Print and shaded views of the part. All mm, measured from the part's lowest x, y and z. A direction names the side the tool comes from. Coordinates: 2 decimals unless noted, no trailing zeros. Loops run counter-clockwise (first coordinate to the right, second up) from the corner with the lowest first, then second, coordinate; pieces in that order, holes last. Notation, with made-up numbers: (14, -2) -> (52, -2) arc R22 ccw to (52, 11) -> close; hole circle Ø7 at (13, 2.5). An arc over 180 degrees is marked (long way). One line per question, with ' | ' between items. Start each with the question number.
1) Probe L1, parallel to Y at x = 9.75, z = 8.5; L2, parallel to Y at x = 1.5, z = 3; L3, parallel to Z at x = 12.25, y = 17.5. List the from-to ranges inside material, lowest first. Write a range as from..to.
2) Cut at A-A (x = 7.05). List the corners of the cut face in (y, z), plus the area to 3 significant figures.
3) Drop flat-ended pins along their axis: pin 1 (2 mm diameter, centred on x = 3, y = 22.5, fed in from +Z); pin 2 (1.5 mm diameter, centred on y = 29, z = 1.5, fed in from +X); pin 3 (4 mm diameter, centred on x = 3.5, y = 34, fed in from +Z). Give the stop position or say it passes through.
4) 3-axis set-ups, long thin cutter, end or side, ignore diameter. For the marked faces 1 and 2: which of +Z, -Z, +X, -X, +Y, -Y reach the whole face in a straight line?
5) Cut at B-B (y = 17). List the corners of the cut face in (x, z), plus the area to 3 significant figures.
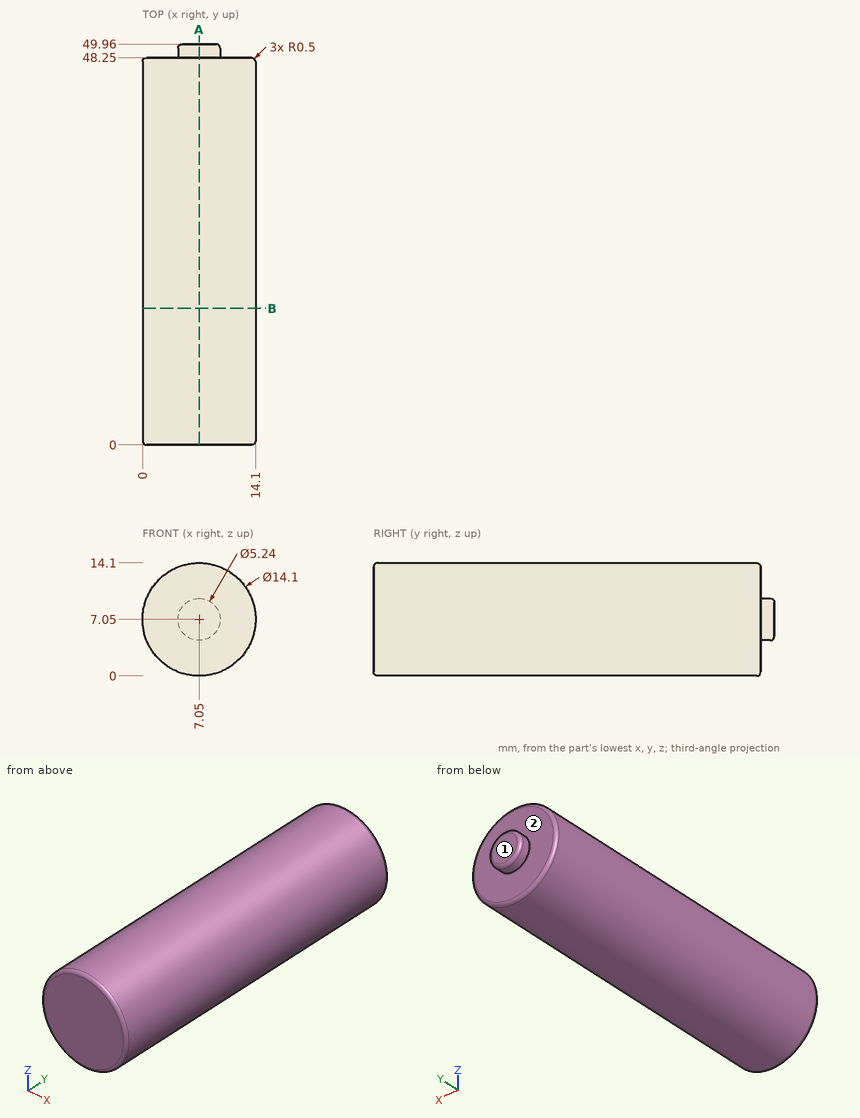
Reported:
1) L1: y = 0..48.25 | L2: y = 0.12..48.13 | L3: z = 2.29..11.81
2) outline: (0, 0.5) arc R0.5 ccw to (0.5, 0) -> (47.75, 0) arc R0.5 ccw to (48.25, 0.5) -> (48.25, 4.43) -> (49.46, 4.43) arc R0.5 ccw to (49.96, 4.93) -> (49.96, 9.17) arc R0.5 ccw to (49.46, 9.67) -> (48.25, 9.67) -> (48.25, 13.6) arc R0.5 ccw to (47.75, 14.1) -> (0.5, 14.1) arc R0.5 ccw to (0, 13.6) -> close | area: 689 mm²
3) pin 1: stops at z = 13.41 | pin 2: stops at x = 12.21 | pin 3: stops at z = 13.93
4) face 1: +Z, -Z, +X, -X, +Y | face 2: +Y
5) outline: circle Ø14.1 at (7.05, 7.05) | area: 156 mm²
